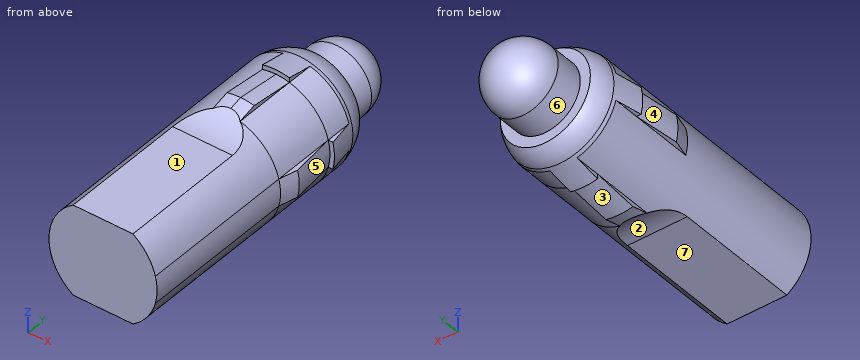
```python
from build123d import *

# Parameters (mm, degrees)
CUT_EXTRUDE1_DEPTH = 39.124795081
CUT_EXTRUDE2_DEPTH = 10


with BuildPart() as part:
    # Sketch2 → Revolve1 (revolve)
    with BuildSketch(Plane.XY, mode=Mode.PRIVATE) as revolve1_sk:
        with BuildLine():
            Line((0, 0), (6, 0))
            Line((6, 0), (6, 17.5))
            Line((6, 17.5), (6.5, 19.5))
            Line((6.5, 19.5), (6, 24.5))
            Line((6, 24.5), (6.5, 24.5))
            Line((6.5, 24.5), (5.928481161, 27.842658555))
            ThreePointArc((5.928481161, 27.842658555), (5.59270884, 28.976619718), (5, 30))
            Line((5, 30), (3.875, 30))
            Line((3.875, 30), (3.875, 33.125))
            ThreePointArc((3.875, 33.125), (2.740038777, 35.865038777), (0, 37))
            Line((0, 37), (0, 0))
        make_face()
    revolve(revolve1_sk.sketch.rotate(Axis((0, 37, 0), (0, -1, 0)), 90), axis=Axis((0, 37, 0), (0, -1, 0)))

    # Sketch3 → Cut-Extrude1 (cut, through all)
    with BuildSketch(Plane.XZ):
        with BuildLine():
            Line((-5.809475019, 1.5), (-7.579692196, 1.5))
            Line((-7.579692196, 1.5), (-7.579692196, 7.495465701))
            Line((-7.579692196, 7.495465701), (-1.5, 7.495465701))
            Line((-1.5, 7.495465701), (-1.5, 5.809475019))
            ThreePointArc((-1.5, 5.809475019), (-4.242640687, 4.242640687), (-5.809475019, 1.5))
        make_face()
        with BuildLine():
            Line((1.5, 7.495465701), (1.5, 5.809475019))
            ThreePointArc((1.5, 5.809475019), (4.242640687, 4.242640687), (5.809475019, 1.5))
            Line((5.809475019, 1.5), (7.579692196, 1.5))
            Line((7.579692196, 1.5), (7.579692196, 7.495465701))
            Line((7.579692196, 7.495465701), (1.5, 7.495465701))
        make_face()
        with BuildLine():
            Line((5.809475019, -1.5), (7.579692196, -1.5))
            Line((7.579692196, -1.5), (7.579692196, -7.495465701))
            Line((7.579692196, -7.495465701), (1.5, -7.495465701))
            Line((1.5, -7.495465701), (1.5, -5.809475019))
            ThreePointArc((1.5, -5.809475019), (4.242640687, -4.242640687), (5.809475019, -1.5))
        make_face()
        with BuildLine():
            Line((-1.5, -7.495465701), (-1.5, -5.809475019))
            ThreePointArc((-1.5, -5.809475019), (-4.242640687, -4.242640687), (-5.809475019, -1.5))
            Line((-5.809475019, -1.5), (-7.579692196, -1.5))
            Line((-7.579692196, -1.5), (-7.579692196, -7.495465701))
            Line((-7.579692196, -7.495465701), (-1.5, -7.495465701))
        make_face()
    extrude(amount=-CUT_EXTRUDE1_DEPTH, mode=Mode.SUBTRACT)

    # Sketch4 → Cut-Extrude2 (cut, symmetric)
    with BuildSketch(Plane(origin=(0, 0, 0), x_dir=(0, 0, -1), z_dir=(1, 0, 0))):
        with BuildLine():
            Line((-5, 0), (-5, 14.110770665))
            ThreePointArc((-5, 14.110770665), (-7.196699141, 19.414071524), (-12.5, 21.610770665))
            Line((-12.5, 21.610770665), (-12.5, 0))
            Line((-12.5, 0), (-5, 0))
        make_face()
        with BuildLine():
            Line((12.5, 0), (5, 0))
            Line((5, 0), (5, 14.110770665))
            ThreePointArc((5, 14.110770665), (7.196699141, 19.414071524), (12.5, 21.610770665))
            Line((12.5, 21.610770665), (12.5, 0))
        make_face()
    extrude(amount=CUT_EXTRUDE2_DEPTH, both=True, mode=Mode.SUBTRACT)


solid = part.part
```
The model under review builds one solid part; all positions refer to its coordinate system, in mm. Face numbers are marked on the shaded views. A direction names the side the tool comes from. Round coordinates to 2 decimals unless told otherwise and drop trailing zeros. Use a Markdown table: item, result.
1) Insertion check: pin 1 (2 mm diameter, centred on x = -1, y = 4.5, fed in from +Z); pin 2 (5 mm diameter, centred on x = 4, y = 11, fed in from -Z); pin 3 (6 mm diameter, centred on x = -4, z = -2.5, fed in from +Y). Each pin has a flat end and moves straight along its axis. Give the tip position at first contact, or say it passes through.
Report:
| item | result |
|---|---|
| pin 1 | z = 5 |
| pin 2 | z = -5 |
| pin 3 | y = 36.6 |
2) Wall thickness on line 1 along Z through (x, y) = (5, 19.5); line 2 along Y through (x, z) = (2.75, -4); line 3 along Z through (x, y) = (2.5, 13.5): over which ranges is each line inside the solid? List them lowest first. Write a range as [from, to].
Report:
| item | result |
|---|---|
| line 1 | [-3.32, 3.32] |
| line 2 | [0, 30] |
| line 3 | [-5, 5] |
3) Draft analysis for pull direction Y (two halves, no side actions). For the marked faces 1, 2, 3 and 4, state which applies: released by +Y, released by -Y, zero draft, split by the parting line, or undercut.
Report:
| item | result |
|---|---|
| face 1 | zero draft |
| face 2 | released by -Y |
| face 3 | undercut |
| face 4 | undercut |
4) Tool access review of the marked faces 5, 6 and 7: name each direction out of +Z, -Z, +X, -X, +Y, -Y from which nothing blocks a thin tool from reaching the whole face with its end or side.
Report:
| item | result |
|---|---|
| face 5 | +X |
| face 6 | +Y |
| face 7 | -Z, +X, -X, -Y |
